from build123d import *

# Parameters (mm, degrees)
BOSS_EXTRUDE2_DEPTH = 65
CUT_EXTRUDE1_DEPTH  = 55
SKETCH4_W           = 26
SKETCH4_H           = 55
CUT_EXTRUDE2_DEPTH  = 17
SKETCH10_W          = 26
SKETCH10_H          = 55
CUT_EXTRUDE3_DEPTH  = 17
SKETCH9_W           = 26
SKETCH9_H           = 55
CUT_EXTRUDE4_DEPTH  = 17
SKETCH8_W           = 26
SKETCH8_H           = 55
CUT_EXTRUDE5_DEPTH  = 17
SKETCH7_W           = 26
SKETCH7_H           = 55
CUT_EXTRUDE6_DEPTH  = 17
SKETCH6_W           = 26
SKETCH6_H           = 55
CUT_EXTRUDE7_DEPTH  = 17
SKETCH11_W          = 7.5
SKETCH11_H          = 15
BOSS_EXTRUDE4_DEPTH = 55
SKETCH12_R          = 1.25
CUT_EXTRUDE8_DEPTH  = 17
SKETCH13_R          = 1.25
CUT_EXTRUDE9_DEPTH  = 11
CUT_EXTRUDE10_START = -11
SKETCH14_R          = 1.25
CUT_EXTRUDE10_DEPTH = 11
SKETCH15_R          = 1.25
CUT_EXTRUDE11_DEPTH = 43
SKETCH16_R          = 1.25
CUT_EXTRUDE12_DEPTH = 43
SKETCH17_R          = 1.25
CUT_EXTRUDE13_DEPTH = 43
SKETCH18_R          = 1.25
CUT_EXTRUDE14_DEPTH = 43
SKETCH19_R          = 1.25
CUT_EXTRUDE15_DEPTH = 43
SKETCH20_R          = 2.5
CUT_EXTRUDE16_DEPTH = 3


with BuildPart() as part:
    # Sketch1 → Boss-Extrude2 (new body)
    with BuildSketch(Plane(origin=(0, 0, 0), x_dir=(1, 0, 0), z_dir=(0, 1, 0))):
        Polygon((-42.489685364, -94.349995431), (41.923987132, -94.349995431), (113.2396696, -1.586008434), (41.923987132, 91.177978564), (-42.489685364, 91.177978564), (-113.805367831, -1.586008434), align=None)
    extrude(amount=BOSS_EXTRUDE2_DEPTH)

    # Sketch5 → Cut-Extrude1 (cut)
    with BuildSketch(Plane(origin=(0, 65, 0), x_dir=(1, 0, 0), z_dir=(0, 1, 0))):
        Polygon((-96.734562657, -1.348107169), (-36.116232559, 77.501281779), (35.635389063, 77.501281779), (96.25371916, -1.348107169), (35.635389063, -80.197496117), (-36.116232559, -80.197496117), align=None)
    extrude(amount=-CUT_EXTRUDE1_DEPTH, mode=Mode.SUBTRACT)

    # Sketch4 → Cut-Extrude2 (cut)
    with BuildSketch(Plane(origin=(-70.762900796, 0, -54.40154878), x_dir=(-0.6094893586708845, 0, 0.792794249264558), z_dir=(-0.7927942492645579, 0, -0.6094893586708844))):
        with Locations((12.116086518, 37.5)):
            Rectangle(SKETCH4_W, SKETCH4_H)
    extrude(amount=-CUT_EXTRUDE2_DEPTH, mode=Mode.SUBTRACT)

    # Sketch10 → Cut-Extrude3 (cut)
    with BuildSketch(Plane(origin=(-72.295618263, 0, 55.579880973), x_dir=(0.6094893586708846, 0, 0.7927942492645578), z_dir=(-0.7927942492645578, 0, 0.6094893586708846))):
        with Locations((-9.601329787, 37.5)):
            Rectangle(SKETCH10_W, SKETCH10_H)
    extrude(amount=-CUT_EXTRUDE3_DEPTH, mode=Mode.SUBTRACT)

    # Sketch9 → Cut-Extrude4 (cut)
    with BuildSketch(Plane.XY.offset(94.349995431)):
        with Locations((-0.282849116, 37.5)):
            Rectangle(SKETCH9_W, SKETCH9_H)
    extrude(amount=-CUT_EXTRUDE4_DEPTH, mode=Mode.SUBTRACT)

    # Sketch8 → Cut-Extrude5 (cut)
    with BuildSketch(Plane(origin=(71.940064072, 0, 55.306535781), x_dir=(0.6094893586708842, 0, -0.7927942492645581), z_dir=(0.7927942492645581, 0, 0.6094893586708842))):
        with Locations((9.256542735, 37.5)):
            Rectangle(SKETCH8_W, SKETCH8_H)
    extrude(amount=-CUT_EXTRUDE5_DEPTH, mode=Mode.SUBTRACT)

    # Sketch7 → Cut-Extrude6 (cut)
    with BuildSketch(Plane(origin=(70.407346604, 0, -54.128203588), x_dir=(-0.6094893586708847, 0, -0.7927942492645578), z_dir=(0.7927942492645579, 0, -0.6094893586708847))):
        with Locations((-11.771299466, 37.5)):
            Rectangle(SKETCH7_W, SKETCH7_H)
    extrude(amount=-CUT_EXTRUDE6_DEPTH, mode=Mode.SUBTRACT)

    # Sketch6 → Cut-Extrude7 (cut)
    with BuildSketch(Plane(origin=(0, 0, -91.177978564), x_dir=(-1, 0, 0), z_dir=(0, 0, -1))):
        with Locations((0.282849116, 37.5)):
            Rectangle(SKETCH6_W, SKETCH6_H)
    extrude(amount=-CUT_EXTRUDE7_DEPTH, mode=Mode.SUBTRACT)

    # Sketch11 → Boss-Extrude4 (add)
    with BuildSketch(Plane(origin=(0, 10, 0), x_dir=(1, 0, 0), z_dir=(0, 1, 0))):
        with Locations((-17.032849116, -72.697496117)):
            Rectangle(SKETCH11_W, SKETCH11_H)
        with Locations((16.467150884, -72.697496117)):
            Rectangle(SKETCH11_W, SKETCH11_H)
        with Locations((-17.032849116, 70.001281779)):
            Rectangle(SKETCH11_W, SKETCH11_H)
        with Locations((16.467150884, 70.001281779)):
            Rectangle(SKETCH11_W, SKETCH11_H)
        Polygon((-75.226545521, -29.324694546), (-63.334631782, -20.182354166), (-67.905801972, -14.236397297), (-79.797715711, -23.378737677), align=None)
        Polygon((-59.379822195, -49.937345027), (-47.487908456, -40.795004647), (-42.916738266, -46.740961516), (-54.808652005, -55.883301897), align=None)
        Polygon((-75.456453141, 26.329427508), (-63.564539402, 17.187087128), (-68.135709592, 11.241130258), (-80.027623331, 20.383470638), align=None)
        Polygon((-59.609729815, 46.942077989), (-47.717816076, 37.799737608), (-43.146645886, 43.745694478), (-55.038559625, 52.888034858), align=None)
        Polygon((58.867457093, -49.978346806), (46.975543354, -40.836006426), (42.404373164, -46.781963295), (54.296286903, -55.924303675), align=None)
        Polygon((74.714180418, -29.365696325), (62.822266679, -20.223355945), (67.393436869, -14.277399075), (79.285350608, -23.419739455), align=None)
        Polygon((74.944088038, 26.370429286), (63.0521743, 17.228088906), (67.62334449, 11.282132037), (79.515258229, 20.424472417), align=None)
        Polygon((59.097364713, 46.983079767), (47.205450974, 37.840739387), (42.634280784, 43.786696257), (54.526194523, 52.929036637), align=None)
    extrude(amount=BOSS_EXTRUDE4_DEPTH)

    # Sketch12 → Cut-Extrude8 (cut)
    with BuildSketch(Plane(origin=(0, 10, 0), x_dir=(1, 0, 0), z_dir=(0, 1, 0))):
        with Locations(Location((-0.282849116, -70.197496117, 0), (0, 0, 270))):
            Circle(SKETCH12_R)
        with Locations(Location((-59.375241365, -33.5361262, 0), (0, 0, 270))):
            Circle(SKETCH12_R)
        with Locations(Location((-59.605148985, 30.540859161, 0), (0, 0, 270))):
            Circle(SKETCH12_R)
        with Locations(Location((-0.282849116, 67.501281779, 0), (0, 0, 270))):
            Circle(SKETCH12_R)
        with Locations(Location((59.092783883, 30.58186094, 0), (0, 0, 270))):
            Circle(SKETCH12_R)
        with Locations(Location((58.862876263, -33.577127979, 0), (0, 0, 270))):
            Circle(SKETCH12_R)
    extrude(amount=-CUT_EXTRUDE8_DEPTH, mode=Mode.SUBTRACT)

    # Sketch13 → Cut-Extrude9 (cut)
    with BuildSketch(Plane(origin=(-13.282849116, 0, 0), x_dir=(0, 0, -1), z_dir=(1, 0, 0))):
        with Locations((67.501281779, 28.4)):
            Circle(SKETCH13_R)
        with Locations((67.501281779, 19.2)):
            Circle(SKETCH13_R)
    extrude(amount=-CUT_EXTRUDE9_DEPTH, mode=Mode.SUBTRACT)

    # Sketch14 → Cut-Extrude10 (cut)
    with BuildSketch(Plane.ZY.offset(-12.717150884).offset(CUT_EXTRUDE10_START)):
        with Locations(Location((-67.501281779, 19.2, 0), (0, 0, 180))):
            Circle(SKETCH14_R)
        with Locations((-67.501281779, 26.82449259)):
            Circle(SKETCH14_R)
    extrude(amount=CUT_EXTRUDE10_DEPTH, mode=Mode.SUBTRACT)

    # Sketch15 → Cut-Extrude11 (cut)
    with BuildSketch(Plane(origin=(-5.320050091, 0, -6.920063587), x_dir=(-0.7927942492645578, 0, 0.6094893586708846), z_dir=(-0.6094893586708846, 0, -0.7927942492645578))):
        with Locations((-65.487738047, 19.2)):
            Circle(SKETCH15_R)
        with Locations((-65.487738047, 28.4)):
            Circle(SKETCH15_R)
    extrude(amount=-CUT_EXTRUDE11_DEPTH, mode=Mode.SUBTRACT)

    # Sketch16 → Cut-Extrude12 (cut)
    with BuildSketch(Plane(origin=(18.136296148, 0, -23.590815958), x_dir=(-0.7927942492645582, 0, -0.6094893586708842), z_dir=(0.6094893586708842, 0, -0.7927942492645582))):
        with Locations((-67.131051994, 28.4)):
            Circle(SKETCH16_R)
        with Locations((-67.131051994, 19.2)):
            Circle(SKETCH16_R)
    extrude(amount=-CUT_EXTRUDE12_DEPTH, mode=Mode.SUBTRACT)

    # Sketch17 → Cut-Extrude13 (cut)
    with BuildSketch(Plane.ZY.offset(20.782849116)):
        with Locations((70.197496117, 19.2)):
            Circle(SKETCH17_R)
        with Locations((70.197496117, 28.4)):
            Circle(SKETCH17_R)
    extrude(amount=-CUT_EXTRUDE13_DEPTH, mode=Mode.SUBTRACT)

    # Sketch18 → Cut-Extrude14 (cut)
    with BuildSketch(Plane(origin=(6.642623519, 0, 8.64040307), x_dir=(0.7927942492645585, 0, -0.6094893586708838), z_dir=(0.6094893586708837, 0, 0.7927942492645584))):
        with Locations((-67.512261953, 19.2)):
            Circle(SKETCH18_R)
        with Locations((-67.512261953, 28.4)):
            Circle(SKETCH18_R)
    extrude(amount=-CUT_EXTRUDE14_DEPTH, mode=Mode.SUBTRACT)

    # Sketch19 → Cut-Extrude15 (cut)
    with BuildSketch(Plane(origin=(5.109906051, 0, -6.646718395), x_dir=(-0.7927942492645588, 0, -0.6094893586708833), z_dir=(0.6094893586708833, 0, -0.7927942492645588))):
        with Locations((65.868948006, 19.2)):
            Circle(SKETCH19_R)
        with Locations((65.868948006, 28.4)):
            Circle(SKETCH19_R)
    extrude(amount=-CUT_EXTRUDE15_DEPTH, mode=Mode.SUBTRACT)

    # Sketch20 → Cut-Extrude16 (cut)
    with BuildSketch(Plane(origin=(0, 65, 0), x_dir=(1, 0, 0), z_dir=(0, 1, 0))):
        with Locations(Location((104.74669438, -1.467057801, 0), (0, 0, 270))):
            Circle(SKETCH20_R)
        with Locations(Location((38.779688098, 84.339630172, 0), (0, 0, 270))):
            Circle(SKETCH20_R)
        with Locations(Location((-39.302958961, 84.339630172, 0), (0, 0, 270))):
            Circle(SKETCH20_R)
        with Locations(Location((-105.269965244, -1.467057801, 0), (0, 0, 270))):
            Circle(SKETCH20_R)
        with Locations(Location((-39.302958961, -87.273745774, 0), (0, 0, 270))):
            Circle(SKETCH20_R)
        with Locations(Location((38.779688098, -87.273745774, 0), (0, 0, 270))):
            Circle(SKETCH20_R)
    extrude(amount=-CUT_EXTRUDE16_DEPTH, mode=Mode.SUBTRACT)


solid = part.part
Geometry check sheet. Reference: the model listing, model coordinates, mm. A direction names the side the tool comes from. Give positions to 0.01 mm unless a question says otherwise; leave off trailing zeros. Loops run counter-clockwise (first coordinate to the right, second up) from the corner with the lowest first, then second, coordinate; pieces in that order, holes last. Notation, with made-up numbers: (-31, 39) -> (-9, 39) arc R22 cw to (-9, 53) -> close; hole circle Ø3 at (-20.5, -24.75). An arc over 180 degrees is marked (long way). Answer in a Markdown table with one row per item. Add a question column.
1) Gauge pin test, flat ends, axial feed: P1, Ø4, axis at x = 78.5, y = 30, coming from the +Z side; P2, Ø12, axis at x = 4, z = -71, coming from the +Y side; P3, Ø2, axis at x = -83, y = 39, coming from the +Z side. Record the tip position at first contact, or that the pin passes through.
2) Cross-section at A-A on x = -25. Record the boundary of the cut face in (y, z), and give its area (3 significant figures).
3) Set-up check for faces 3 (the face through (-95, 65, 9)), 4 (the face through (20.217, 37, 73)): record each of +Z, -Z, +X, -X, +Y, -Y from which the full face is reachable in a straight line by a thin tool's end or side.
4) Draft check along X on faces 1 (the face through (-39, 62, -84)), 2 (the face through (93, 65, -7)). Enter one of: pulls with the +X half, pulls with the -X half, needs draft (parallel to the pull), parting line crosses it, or undercut.
5) Material ranges on probe 1 along Z at (x, y) = (48, 12); probe 2 along Z at (x, y) = (-45, 54.5); probe 3 along Z at (x, y) = (13.5, 60), recorded low to high. Write a range as from..to.
6) Cross-section at B-B on y = 44. State how many separate pieces and enclosed holes the cut face has, and give its area (3 significant figures).
Outcome:
| question | item | result |
|---|---|---|
| 1 | P1 | stops at z = 33.81 |
| 1 | P2 | stops at y = 10 |
| 1 | P3 | stops at z = 36.07 |
| 2 | outline | (0, -91.18) -> (65, -91.18) -> (65, -77.5) -> (10, -77.5) -> (10, 80.2) -> (65, 80.2) -> (65, 94.35) -> (0, 94.35) -> close |
| 2 | area | 3,390 mm^2 |
| 3 | face 3 | +Z, -Z, +X, -X, +Y |
| 3 | face 4 | +Y |
| 4 | face 1 | undercut |
| 4 | face 2 | needs draft |
| 5 | probe 1 | z = -83.27..-61.42, -47.91..-38.45, 41.62..51.08, 64.11..86.45 |
| 5 | probe 2 | z = -87.91..-65.95, -45.17..-41.33, 44.03..48.34, 68.64..91.08 |
| 5 | probe 3 | z = -91.18..-62.5, 65.2..94.35 |
| 6 | separate pieces | 6 |
| 6 | enclosed holes | 0 |
| 6 | area | 7,240 mm^2 |
